Can you work these out from the model? Positions are in its coordinate system, mm. Round coordinates to 2 decimals unless told otherwise and drop trailing zeros. Write each loop counter-clockwise with the first axis right and the second up, starting at its lowest first coordinate (ties: lowest second). Pieces come first, ordered by that corner, then holes. Notation, with made-up numbers: (-9.75, -19) -> (40.25, -19) arc R12 ccw to (40.25, -4) -> close; hole circle Ø6 at (-31, -20). An arc over 180 degrees is marked (long way). Use CSV: the item, a comma, the result in double quotes.
Autodesk Inventor part; units mm, degrees
ref_plane "YZ Plane" through (0, 0, 0) normal (1, 0, 0) x (0, 1, 0)
ref_plane "XZ Plane" through (0, 0, 0) normal (0, 1, 0) x (-1, 0, 0)
ref_plane "XY Plane" through (0, 0, 0) normal (0, 0, 1) x (1, 0, 0)
sketch "Sketch1" plane through (0, 0, 0) normal (0, 1, 0) x (-1, 0, 0)
  line L0 (0, 0) -> (100, 0)
  line L1 (100, 0) -> (100, -20)
  line L2 (100, -20) -> (0, -20)
  line L3 (0, -20) -> (0, 0)
  circle A0 centre (95, -10) radius 2.75
  circle A1 centre (5, -10) radius 2.75
  point P0 (0, -10)
  point P1 (100, -10)
  dimension "d0" = 20
  dimension "d1" = 100
  dimension "d2" = 5.5
  dimension "d3" = 5.5
  dimension "d4" = 5
  dimension "d5" = 5
extrude "Extrusion1" add sketch "Sketch1" along normal blind 5
sketch "Sketch2" plane through (0, 0, 0) normal (0, -1, 0) x (1, 0, 0)
  circle A0 centre (-19.165, -10) radius 2.75
  circle A1 centre (-5, -10) radius 2.75
  line L0 (-100, 0) -> (0, 0)
  dimension "d8" = 5.5
  dimension "d9" = 14.165
  dimension "d10" = 10
extrude "Extrusion2" cut sketch "Sketch2" against normal blind 10 contours A0
properties part number "RollYAxis" material "Wood (Birch)"
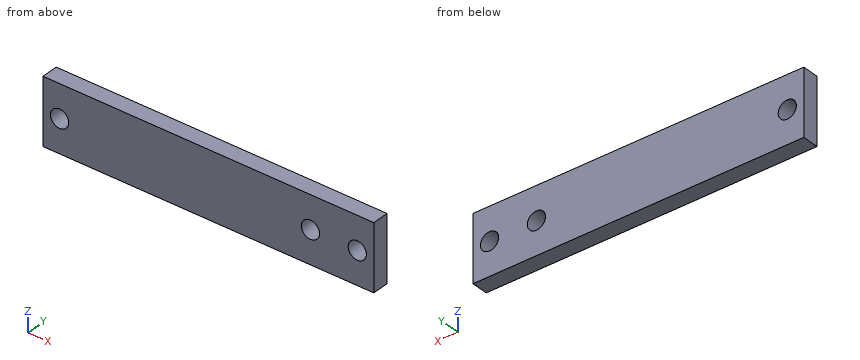
Q1. Please list where these lines run through material, in increasing order: probe 1 along Z at (x, y) = (-5, 3.35); probe 2 along X at (y, z) = (2.55, -9.5); probe 3 along Z at (x, y) = (-93, 2.65).
Resolved:
probe 1,"z = -20 to -12.75, -7.25 to 0"
probe 2,"x = -100 to -97.7, -92.3 to -21.87, -16.46 to -7.7, -2.3 to 0"
probe 3,"z = -20 to -11.89, -8.11 to 0"
Q2. Will this pin go through, and if not, where does the flat tip stop? P1, Ø9, axis at x = -19.165, z = -10, coming from the +Y side.
Resolved:
P1,"stops at y = 5"
Q3. Suppose I cut it at A-A (z = -10). Write out the boundary of the cut face in (x, y) (3 decimals).
Resolved:
outline,"(-100, 0) -> (-97.75, 0) -> (-97.75, 5) -> (-100, 5) -> close; (-92.25, 0) -> (-21.915, 0) -> (-21.915, 5) -> (-92.25, 5) -> close; (-16.415, 0) -> (-7.75, 0) -> (-7.75, 5) -> (-16.415, 5) -> close; (-2.25, 0) -> (0, 0) -> (0, 5) -> (-2.25, 5) -> close"
Q4. Suppose I cut it at C-C (x = -5). Write out the boundary of the cut face in (y, z).
Resolved:
outline,"(0, -20) -> (5, -20) -> (5, -12.75) -> (0, -12.75) -> close; (0, -7.25) -> (5, -7.25) -> (5, 0) -> (0, 0) -> close"
Q5. Suppose I cut it at B-B (y = 2.4). Write out the boundary of the cut face in (x, z) (3 decimals).
Resolved:
outline,"(-100, -20) -> (0, -20) -> (0, 0) -> (-100, 0) -> close; hole circle Ø5.5 at (-95, -10); hole circle Ø5.5 at (-19.165, -10); hole circle Ø5.5 at (-5, -10)"
